```python
from build123d import *

# Parameters (mm, degrees)
F1_DEPTH = 6.35
F3_DEPTH = 3.175


with BuildPart() as f1:
    # F0 (on Top) → F1 (new body)
    with BuildSketch(Plane.XY):
        Polygon((-177.8, 0), (0, 0), (0, 139.7), (-25.4, 139.7), (-25.4, 25.4), (-177.8, 25.4), align=None)
    extrude(amount=F1_DEPTH)

    # F2 (on face) → F3 (cut)
    with BuildSketch(Plane.XY.offset(6.35)):
        Polygon((-177.8, 25.4), (-177.8, 12.7), (-25.4, 12.7), (-12.7, 12.7), (-12.7, 25.4), (-12.7, 139.7), (-25.4, 139.7), (-25.4, 25.4), align=None)
    extrude(amount=-F3_DEPTH, mode=Mode.SUBTRACT)


solid = f1.part
```
Geometry check sheet. Reference: the model listing, model coordinates, mm. A direction names the side the tool comes from. Coordinates: 2 decimals unless noted, no trailing zeros. Order: outer loops, then holes, each group sorted by start corner. A loop starts at its lowest first (then second) coordinate and runs counter-clockwise, first axis right, second up. Notation, with made-up numbers: M 2.25,-7.5 L 50.25,-7.5 A14 cw 50.25,1.5 Z; hole C -14,35.5 d11. An arc over 180 degrees is marked long. Answer as a JSON object with one key per item and string values.
Q1. Cross-section at B-B on z = 1. Record the cut outline in (x, y), and give its area (3 significant figures).
Results are:
{"outline": "M -177.8,0 L 0,0 L 0,139.7 L -25.4,139.7 L -25.4,25.4 L -177.8,25.4 Z", "area": "7,420 mm²"}
Q2. Tool access check on faces 1 (the flat face through (-65, 25, 3.175)), 2 (the flat face through (-177.8, 10, 2)). Record the directions out of +Z, -Z, +X, -X, +Y, -Y that give a thin tool (end or side, any length) a straight path to the whole face; none if there is none.
Results are:
{"face 1": "+Z, -X, +Y", "face 2": "+Z, -Z, -X, +Y, -Y"}
Q3. Cross-section at A-A on x = -15.5. Record the cut outline in (y, z) (3 decimals), and give its area (3 significant figures).
Results are:
{"outline": "M 0,0 L 139.7,0 L 139.7,3.175 L 12.7,3.175 L 12.7,6.35 L 0,6.35 Z", "area": "484 mm²"}
Q4. Scan lines: line 1 (X direction, y = 37, z = 6.25); line 2 (Y direction, x = -73, z = 5.5); line 3 (Y direction, x = -27, z = 1). Record each from-to range of solid material in increasing order.
Results are:
{"line 1": "x = -12.7 to 0", "line 2": "y = 0 to 12.7", "line 3": "y = 0 to 25.4"}
Q5. Depth check by flat-ended pin: pin 1 Ø1 at (y, z) = (69, 1.5) entering from -X; pin 2 Ø1.6 at (x, z) = (-74, 1.5) entering from +Y; pin 3 Ø2 at (y, z) = (83, 5.5) entering from -X. Enter the tip coordinate at first touch or a pass-through.
Results are:
{"pin 1": "stops at x = -25.4", "pin 2": "stops at y = 25.4", "pin 3": "stops at x = -12.7"}
